Autodesk Inventor part; units mm, degrees
ref_plane "Work Plane1" through (0, 0, 2.5241) normal (0, 0, 1) x (1, 0, 0)
ref_plane "YZ Plane" through (0, 0, 0) normal (1, 0, 0) x (0, 1, 0)
ref_plane "XZ Plane" through (0, 0, 0) normal (0, 1, 0) x (-1, 0, 0)
ref_plane "Work Plane1" through (0, 0, 2.5241) normal (0, 0, 1) x (1, 0, 0)
sketch "Sketch1" plane through (0, 0, 2.5241) normal (0, 0, 1) x (1, 0, 0)
  line L0 (-4, 272) -> (-4, -8) construction
  line L1 (4, 272) -> (4, -8) construction
  line L2 (76, 272) -> (76, -8) construction
  line L3 (84, 272) -> (84, -8) construction
  line L4 (84, -8) -> (-4, -8) construction
  line L5 (84, 106) -> (80, 106) construction
  line L6 (80, 110) -> (76, 110) construction
  line L7 (-3.365, 272) -> (-3.365, -7.365) construction
  line L8 (-3.365, -7.365) -> (83.365, -7.365) construction
  line L9 (83.365, -7.365) -> (83.365, 272) construction
  line L10 (-3.365, -7.365) -> (83.365, -7.365)
  line L11 (83.365, -7.365) -> (83.365, 107.95)
  line L12 (-3.365, 107.95) -> (-3.365, -7.365)
  circle A0 centre (0, 12) radius 2
  circle A1 centre (80, 12) radius 2
  circle A2 centre (0, 84) radius 2
  circle A3 centre (80, 84) radius 2
  line L13 (21.39, 107.95) -> (21.39, 11.177)
  line L14 (21.39, 11.177) -> (67.11, 11.177)
  line L15 (67.11, 11.177) -> (67.11, 107.95)
  line L16 (83.365, 107.95) -> (67.11, 107.95)
  line L17 (21.39, 107.95) -> (-3.365, 107.95)
  point P0 (0, 0)
  dimension "d0" = 0.635
  dimension "d1" = 8.89
  dimension "d2" = 45.72
  dimension "d18" = 18.542
extrude "Extrusion1" add sketch "Sketch1" along normal blind 10.16
sketch "Sketch2" plane through (0, 0, 12.6841) normal (0, 0, 1) x (1, 0, 0)
  line L0 (83.365, 107.95) -> (67.11, 107.95)
  line L1 (83.365, -7.365) -> (83.365, 107.95)
  line L2 (67.11, 107.95) -> (83.365, 107.95)
  line L3 (83.365, 107.95) -> (83.365, 23.8125)
  line L4 (67.11, 23.8125) -> (67.11, 107.95)
  circle A0 centre (80, 84) radius 2
  circle A1 centre (80, 84) radius 1.9939
  line L5 (83.365, 23.8125) -> (83.365, -7.365)
  line L6 (83.365, -7.365) -> (67.11, -7.365)
  line L7 (67.11, -7.365) -> (67.11, 23.8125)
  point P0 (0, 0)
  dimension "d5" = 3.9878
extrude "Extrusion2" add sketch "Sketch2" along normal blind 2.54 contours L1 L6 L7 L4 L0
fillet "Fillet1" radius 25.4 1 edges at (75.2375, 107.95, 15.2241)
sketch "Sketch3" plane through (0, 0, 12.6841) normal (0, 0, 1) x (1, 0, 0)
  circle A0 centre (0, 12) radius 2 construction
  circle A1 centre (0, 12) radius 4.8768 construction
  circle A2 centre (0, 84) radius 2 construction
  circle A3 centre (0, 84) radius 4.8768 construction
  circle A4 centre (80, 12) radius 2 construction
  line L0 (0, 16.8768) -> (4.2234, 14.4384)
  line L1 (4.2234, 14.4384) -> (4.2234, 9.5616)
  line L2 (4.2234, 9.5616) -> (0, 7.1232)
  line L3 (0, 7.1232) -> (-4.2234, 9.5616)
  line L4 (-4.2234, 9.5616) -> (-4.2234, 14.4384)
  line L5 (-4.2234, 14.4384) -> (0, 16.8768)
  line L6 (0, 88.8768) -> (4.2234, 86.4384)
  line L7 (4.2234, 86.4384) -> (4.2234, 81.5616)
  line L8 (4.2234, 81.5616) -> (0, 79.1232)
  line L9 (0, 79.1232) -> (-4.2234, 81.5616)
  line L10 (-4.2234, 81.5616) -> (-4.2234, 86.4384)
  line L11 (-4.2234, 86.4384) -> (0, 88.8768)
  point P0 (0, 0)
  dimension "d9" = 9.7536
  dimension "d10" = 9.7536
extrude "Extrusion3" cut sketch "Sketch3" against normal blind 4.826
sketch "Sketch4" plane through (0, 0, 15.2241) normal (0, 0, 1) x (1, 0, 0)
  circle A0 centre (80, 84) radius 2 construction
  circle A1 centre (80, 84) radius 4.8768 construction
  line L0 (80, 88.8768) -> (84.2234, 86.4384)
  line L1 (84.2234, 86.4384) -> (84.2234, 81.5616)
  line L2 (84.2234, 81.5616) -> (80, 79.1232)
  line L3 (80, 79.1232) -> (75.7766, 81.5616)
  line L4 (75.7766, 81.5616) -> (75.7766, 86.4384)
  line L5 (75.7766, 86.4384) -> (80, 88.8768)
  point P0 (0, 0)
  dimension "d14" = 9.7536
extrude "Extrusion4" cut sketch "Sketch4" against normal blind 4.826
sketch "Sketch5" plane through (0, 0, 12.6841) normal (0, 0, 1) x (1, 0, 0)
  line L0 (-3.365, -7.365) -> (67.11, -7.365)
  line L1 (-3.365, -7.365) -> (67.11, -7.365)
  line L2 (67.11, 5.335) -> (-3.365, 5.335)
  line L3 (-3.365, 5.335) -> (-3.365, -7.365)
  line L4 (67.11, 5.335) -> (67.11, -7.365)
  line L5 (-3.365, -7.365) -> (83.365, -7.365)
  point P0 (0, 0)
extrude "Extrusion5" cut sketch "Sketch5" against normal blind 5.08
sketch "Sketch13" plane through (83.365, -7.365, 15.2241) normal (1, 0, 0) x (0, 0, -1)
  line L0 (0, 0) -> (7.62, 0)
  line L1 (0, 0) -> (-10.16, 0)
  line L2 (0, 93.318) -> (0, 0)
  line L3 (0, 0) -> (0, 60.96)
  line L4 (0, 60.96) -> (-10.16, 0)
  point P0 (15.2241, 7.365)
  dimension "d54" = 10.16
  dimension "d55" = 60.96
extrude "Extrusion13" add sketch "Sketch13" against normal blind 6.35
sketch "Sketch14" plane through (0, 0, 15.2241) normal (0, 0, 1) x (1, 0, 0)
  line L0 (67.11, -7.365) -> (77.015, -7.365)
  line L1 (77.015, -7.365) -> (77.015, 53.595)
  line L2 (67.11, -7.365) -> (77.015, -7.365)
  line L3 (77.015, -7.365) -> (77.015, 5.3272)
  line L4 (77.015, 5.3272) -> (67.11, 5.3272)
  line L5 (67.11, 5.3272) -> (67.11, -7.365)
  point P0 (0, 0)
extrude "Extrusion14" cut sketch "Sketch14" against normal up to surface (7.62 mm away)
sketch "Sketch15" plane through (21.39, 11.177, 2.5241) normal (1, 0, 0) x (0, 0, -1)
  line L0 (0, 0) -> (-10.16, 0)
  line L1 (0, 0) -> (-10.16, 0)
  line L2 (0, 0) -> (0, 12.065)
  line L3 (-10.16, 0) -> (-10.16, 96.773)
  line L4 (0, 12.065) -> (-10.16, 0)
  point P0 (2.5241, -11.177)
  dimension "d60" = 12.065
extrude "Extrusion15" add sketch "Sketch15" along normal up to next
equation "\"d61\" = d60"
properties part number "Back Wall with slant"
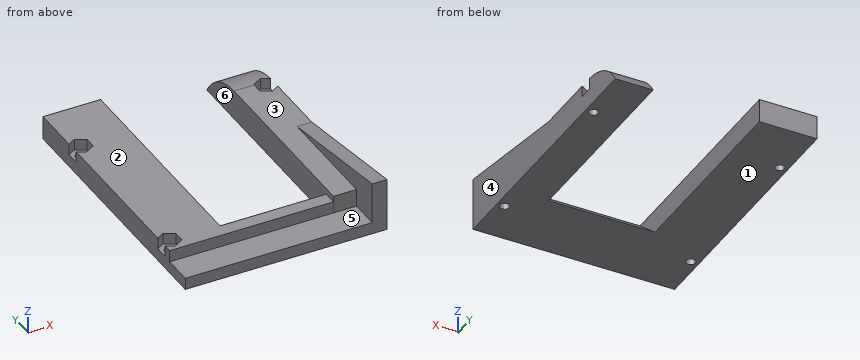
Can you work these out from the model? Positions are in its coordinate system, mm. Face numbers are marked on the shaded views. A direction names the side the tool comes from. Round coordinates to 2 decimals unless told otherwise and drop trailing zeros. Loops run counter-clockwise (first coordinate to the right, second up) from the corner with the lowest first, then second, coordinate; pieces in that order, holes last. Notation, with made-up numbers: (38.25, 69) -> (86.25, 69) arc R24 ccw to (86.25, 79) -> close; hole circle Ø5 at (77, -6). An arc over 180 degrees is marked (long way). Answer in a Markdown table with one row per item.
Item 1: We'd pull the mould along X, two halves only. Please class the marked faces 4, 5 and 6: released by +X, released by -X, zero draft, split by the parting line, or undercut.
Answer block:
| item | result |
|---|---|
| face 4 | released by +X |
| face 5 | zero draft |
| face 6 | undercut |
Item 2: If I drill on probe 1 along Y at (x, z) = (0, 6.35) (3 decimals); probe 2 along X at (y, z) = (84, 6.2) (3 decimals); probe 3 along Z at (x, y) = (14, 49.5), over which ranges is the centre line in solid material (lowest first)?
Answer block:
| item | result |
|---|---|
| probe 1 | -7.365 to 10, 14 to 82, 86 to 107.95 |
| probe 2 | -3.365 to -2, 2 to 21.39, 67.11 to 78, 82 to 83.365 |
| probe 3 | 2.52 to 12.68 |
Item 3: Suppose I cut it at C-C, the plane y = 40.5. List the corners of the cut face in (x, z) for me (3 decimals), plus the area to 3 significant figures.
Answer block:
| item | result |
|---|---|
| outline | (-3.365, 2.524) -> (21.39, 2.524) -> (21.39, 12.684) -> (-3.365, 12.684) -> close; (67.11, 2.524) -> (83.365, 2.524) -> (83.365, 17.407) -> (77.015, 17.407) -> (77.015, 15.224) -> (67.11, 15.224) -> close |
| area | 472 mm² |
Item 4: Will these pins go through, and if not, where does the flat tip stop? P1, Ø1.5, axis at x = 52.5, z = 5.5, coming from the +Y side; P2, Ø3.5, axis at x = 0, y = 84, coming from the +Z side; P3, Ø6, axis at x = 73, z = 12, coming from the -Y side; P4, Ø5.5, axis at y = 84, z = 11, coming from the -X side.
Answer block:
| item | result |
|---|---|
| P1 | y = 20.6 |
| P2 | through |
| P3 | y = 5.33 |
| P4 | x = 3.68 |
Item 5: Suppose I cut it at B-B, the plane x = 36. List the corners of the cut face in (y, z) for me (3 decimals).
Answer block:
| item | result |
|---|---|
| outline | (-7.365, 2.524) -> (23.242, 2.524) -> (11.177, 12.684) -> (5.335, 12.684) -> (5.335, 7.604) -> (-7.365, 7.604) -> close |
Item 6: On a 3-axis mill with a long thin cutter (end or side, diameter ignored), from which of +Z, -Z, +X, -X, +Y, -Y can I reach the whole of each face in a straight line? I mean the marked faces 1, 2 and 3. Say none if no direction works.
Answer block:
| item | result |
|---|---|
| face 1 | -Z, +X, -X, +Y, -Y |
| face 2 | +Z, -X, +Y, -Y |
| face 3 | +Z, -X, +Y |
Item 7: Suppose I cut it at A-A, the plane y = 84. List the corners of the cut face in (x, z) for me (3 decimals), plus the area to 3 significant figures.
Answer block:
| item | result |
|---|---|
| outline | (-3.365, 2.524) -> (-2, 2.524) -> (-2, 7.858) -> (-3.365, 7.858) -> close; (2, 2.524) -> (21.39, 2.524) -> (21.39, 12.684) -> (4.223, 12.684) -> (4.223, 7.858) -> (2, 7.858) -> close; (67.11, 2.524) -> (78, 2.524) -> (78, 10.398) -> (75.777, 10.398) -> (75.777, 15.224) -> (67.11, 15.224) -> close; (82, 2.524) -> (83.365, 2.524) -> (83.365, 10.398) -> (82, 10.398) -> close |
| area | 332 mm² |
Item 8: Suppose I cut it at D-D, the plane y = 21. List the corners of the cut face in (x, z) for me (3 decimals), plus the area to 3 significant figures.
Answer block:
| item | result |
|---|---|
| outline | (-3.365, 2.524) -> (83.365, 2.524) -> (83.365, 20.657) -> (77.015, 20.657) -> (77.015, 15.224) -> (67.11, 15.224) -> (67.11, 4.412) -> (21.39, 4.412) -> (21.39, 12.684) -> (-3.365, 12.684) -> close |
| area | 579 mm² |
